Verification items for the finished model (mm, model axes). A direction names the side the tool comes from. Round coordinates to 2 decimals unless told otherwise and drop trailing zeros. Order: outer loops, then holes, each group sorted by start corner. A loop starts at its lowest first (then second) coordinate and runs counter-clockwise, first axis right, second up. Notation, with made-up numbers: (14.5, 34.5) -> (56.5, 34.5) arc R20 ccw to (56.5, 70.5) -> close; hole circle Ø6 at (-27.75, 31.25). An arc over 180 degrees is marked (long way). Put each result on its own line as item: value.
from build123d import *

# Parameters (mm, degrees)
F1_DEPTH = 3.81
F2_R     = 2.367737602
F3_R     = 0.8284878815
F4_R     = 1.016


with BuildPart() as f1:
    # F0 (on Top) → F1 (new body)
    with BuildSketch(Plane.XY):
        with BuildLine():
            Line((98.3983673645, -11.43), (99.06, -11.43))
            Line((99.06, -11.43), (114.808, -11.43))
            Line((114.808, -11.43), (114.808, 5.842))
            add(Edge.make_bspline(
                [(111.8424964318, 25.4789244169), (114.050069317, 19.269012489), (114.16942194, 10.4852159403), (114.808, 5.842)],
                knots=[0.6566118261, 0.6566118261, 0.6566118261, 0.6566118261, 1, 1, 1, 1], degree=3))
            add(Edge.make_bspline(
                [(95.2225835996, 27.3046364672), (95.2454386696, 29.8195688516), (95.6622303832, 33.3481063354), (104.8322806826, 36.1190012322), (110.1233601043, 30.3148622281), (111.8424964318, 25.4789244169)],
                knots=[0, 0, 0, 0, 0.1826926903, 0.3892000055, 0.6566118261, 0.6566118261, 0.6566118261, 0.6566118261], degree=3))
            ThreePointArc((95.2225835996, 27.3046364672), (95.4714110254, 26.4214548581), (95.7120472042, 25.5360063436))
            Line((95.7120472042, 25.5360063436), (101.4981578414, 23.3149265672))
            Line((101.4981578414, 23.3149265672), (101.7785107441, 21.99596986))
            Line((101.7785107441, 21.99596986), (96.8953013287, 20.5957320924))
            ThreePointArc((96.8953013287, 20.5957320924), (97.0819149886, 19.6973445455), (97.2601992237, 18.7972670078))
            Line((97.2601992237, 18.7972670078), (102.8772804931, 16.1779789954))
            Line((102.8772804931, 16.1779789954), (103.0649447013, 14.8426787705))
            Line((103.0649447013, 14.8426787705), (98.0959548895, 13.7864873811))
            ThreePointArc((98.0959548895, 13.7864873811), (98.2194456206, 12.8772707503), (98.3345093292, 11.9669492766))
            Line((98.3345093292, 11.9669492766), (103.7551953754, 8.9622139361))
            Line((103.7551953754, 8.9622139361), (103.8492566079, 7.617075642))
            Line((103.8492566079, 7.617075642), (98.8186948187, 6.9100762891))
            ThreePointArc((98.8186948187, 6.9100762891), (98.8784103809, 5.9952948679), (98.9296578383, 5.08))
            Line((98.9296578383, 5.08), (104.1276253753, 1.956746008))
            Line((104.1276253753, 1.956746008), (104.1276253753, 0.3543628866))
            Line((104.1276253753, 0.3543628866), (99.06, 0))
            ThreePointArc((99.06, 0), (98.8944535126, -5.7245667466), (98.3983673645, -11.43))
        make_face()
        with BuildLine():
            Line((80.01, -11.43), (98.3983673645, -11.43))
            ThreePointArc((98.3983673645, -11.43), (98.8944535126, -5.7245667466), (99.06, 0))
            Line((99.06, 0), (80.01, -11.43))
        make_face()
        with BuildLine():
            add(Edge.make_bspline(
                [(111.8424964318, 25.4789244169), (114.050069317, 19.269012489), (114.16942194, 10.4852159403), (114.808, 5.842)],
                knots=[0.6566118261, 0.6566118261, 0.6566118261, 0.6566118261, 1, 1, 1, 1], degree=3))
            Line((114.808, 5.842), (129.4839402923, 4.5580215978))
            Line((129.4839402923, 4.5580215978), (111.8424964318, 25.4789244169))
        make_face()
    extrude(amount=F1_DEPTH)

    # F2
    f2_edges = [f1.edges().sort_by_distance(p)[0] for p in [
        (80.01, -11.43, 1.905),
        (129.48394, 4.558022, 1.905),
    ]]
    fillet(f2_edges, radius=F2_R)

    # F3
    f3_edges = [f1.edges().sort_by_distance(p)[0] for p in [
        (104.127625, 0.354363, 1.905),
        (104.127625, 1.956746, 1.905),
        (103.849257, 7.617076, 1.905),
        (103.755195, 8.962214, 1.905),
        (103.064945, 14.842679, 1.905),
        (102.87728, 16.177979, 1.905),
        (101.778511, 21.99597, 1.905),
        (101.498158, 23.314927, 1.905),
        (95.712047, 25.536006, 1.905),
    ]]
    fillet(f3_edges, radius=F3_R)

    # F4
    f4_edges = [f1.edges().sort_by_distance(p)[0] for p in [
        (98.818695, 6.910076, 1.905),
        (98.095955, 13.786487, 1.905),
        (96.895301, 20.595732, 1.905),
        (97.260199, 18.797267, 1.905),
        (98.334509, 11.966949, 1.905),
        (98.929658, 5.08, 1.905),
    ]]
    fillet(f4_edges, radius=F4_R)


solid = f1.part
Item 1: Section check A-A on y = -1.5. Record the boundary of the cut face in (x, z), then the cut area to 3 significant figures.
Check sheet entries:
outline: (96.56, 0) -> (114.81, 0) -> (114.81, 3.81) -> (96.56, 3.81) -> close
area: 69.5 mm^2
Item 2: Material ranges on L1, parallel to Y at x = 99.5, z = 2.75; L2, parallel to Y at x = 100.5, z = 1.2; L3, parallel to X at y = -9, z = 0.2, recorded low to high. Write a range as [from, to].
Check sheet entries:
L1: y = [-11.43, 0.03], [4.74, 6.97], [11.32, 14.08], [17.75, 21.34], [24.08, 34.22]
L2: y = [-11.43, 0.1], [4.14, 7.15], [10.77, 14.3], [17.29, 21.63], [23.7, 34.45]
L3: x = [86.19, 114.81]
Item 3: Section check B-B on x = 116.5. Record the boundary of the cut face in (y, z).
Check sheet entries:
outline: (5.69, 0) -> (19.96, 0) -> (19.96, 3.81) -> (5.69, 3.81) -> close
Item 4: Tool access check on faces 5 (the flat face through (101, -11.43, 2)), 6 (the flat face through (100.066, 17.489, 1.878)). Record the directions out of +Z, -Z, +X, -X, +Y, -Y that give a thin tool (end or side, any length) a straight path to the whole face; none if there is none.
Check sheet entries:
face 5: +Z, -Z, +X, -X, -Y
face 6: +Z, -Z, -X
Item 5: Release check for a two-part mould opening along X. For faces 1 (the flat face through (118.91, 17.1, 1.88)), 2 (the flat face through (101.239, 0.152, 1.878)), 3 (the flat face through (119.226, 5.455, 1.878)), 4 (the flat face through (106, 7, 3.81)) record: +X half, -X half, draft (parallel to the pull), parting line (faces both ways), or undercut.
Check sheet entries:
face 1: +X half
face 2: -X half
face 3: undercut
face 4: draft
